Work out the finished part from the listing and answer in its coordinate system (mm). Face numbers are marked on the shaded views. A direction names the side the tool comes from. Give positions to 0.01 mm unless a question says otherwise; leave off trailing zeros. Write each loop counter-clockwise with the first axis right and the second up, starting at its lowest first coordinate (ties: lowest second). Pieces come first, ordered by that corner, then holes. Notation, with made-up numbers: (67, -28.75) -> (86, -28.75) arc R22 cw to (86, -8.75) -> close; hole circle Ø8 at (72.5, 68.25). An arc over 180 degrees is marked (long way). Use a Markdown table: item, result. Add a question column.
Q1. Section A-A, the plane x = 16.75 is taken. Give the vertices of the cut face in (y, z).
Q2. Consider line 1 (Y direction, x = 0.8, z = 10); line 2 (Y direction, x = 20.75, z = 20). Determine where each line is inside the solid, lowest interval first.
Q3. Each of these flat-tipped pins is pushed along its axis until it touches: pin 1 Ø1 at (x, z) = (19, 28) entering from +Y; pin 2 Ø9.5 at (y, z) = (11.5, 27) entering from +X. Where does it stop, or does it pass through?
Q4. For the marked faces 1 and 2, determine the directions among +Z, -Z, +X, -X, +Y, -Y from which every point of the face is accessible in a straight line to the end or side of a thin tool.
Q5. Section B-B, the plane z = 10 is taken. Give the vertices of the cut face in (x, y).
Q6. Section C-C, the plane y = 15 is taken. Give the vertices of the cut face in (x, z), plus the area to 3 significant figures.
Q7. Section D-D, the plane z = 30 is taken. Give the vertices of the cut face in (x, y).
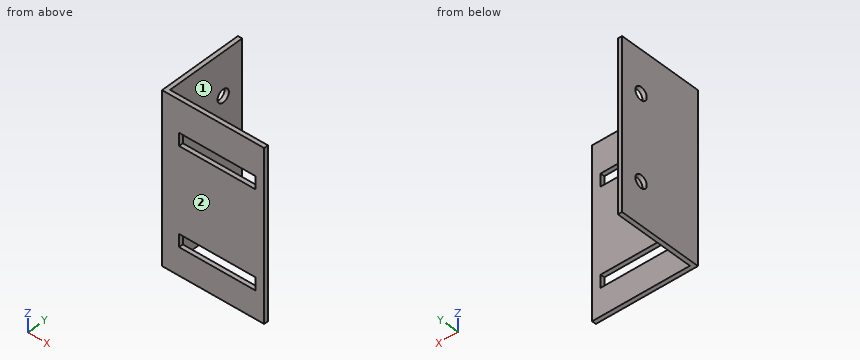
from build123d import *

# Parameters (mm, degrees)
BOSS_EXTRUDE1_DEPTH = 40
SKETCH2_W           = 18
SKETCH2_H           = 3
CUT_EXTRUDE1_DEPTH  = 10
SKETCH3_R           = 1.5
CUT_EXTRUDE2_DEPTH  = 10


with BuildPart() as part:
    # Sketch1 → Boss-Extrude1 (new body)
    with BuildSketch(Plane.XY):
        Polygon((0, 0), (24, 0), (24, 1), (1, 1), (1, 20), (0, 20), align=None)
    extrude(amount=BOSS_EXTRUDE1_DEPTH)

    # Sketch2 → Cut-Extrude1 (cut)
    with BuildSketch(Plane(origin=(0, 1, 0), x_dir=(1, 0, 0), z_dir=(0, 1, 0))):
        with Locations((13, -8)):
            Rectangle(SKETCH2_W, SKETCH2_H)
        with Locations((13, -31)):
            Rectangle(SKETCH2_W, SKETCH2_H)
    extrude(amount=-CUT_EXTRUDE1_DEPTH, mode=Mode.SUBTRACT)

    # Sketch3 → Cut-Extrude2 (cut)
    with BuildSketch(Plane.ZY):
        with Locations((30, 15)):
            Circle(SKETCH3_R)
        with Locations((10, 15)):
            Circle(SKETCH3_R)
    extrude(amount=-CUT_EXTRUDE2_DEPTH, mode=Mode.SUBTRACT)


solid = part.part
Result set:
| question | item | result |
|---|---|---|
| 1 | outline | (0, 0) -> (1, 0) -> (1, 6.5) -> (0, 6.5) -> close; (0, 9.5) -> (1, 9.5) -> (1, 29.5) -> (0, 29.5) -> close; (0, 32.5) -> (1, 32.5) -> (1, 40) -> (0, 40) -> close |
| 2 | line 1 | y = 0 to 13.5, 16.5 to 20 |
| 2 | line 2 | y = 0 to 1 |
| 3 | pin 1 | stops at y = 1 |
| 3 | pin 2 | stops at x = 1 |
| 4 | face 1 | +Z, -Z, +X, +Y |
| 4 | face 2 | +Z, -Z, +X, -X, -Y |
| 5 | outline | (0, 0) -> (24, 0) -> (24, 1) -> (1, 1) -> (1, 13.5) -> (0, 13.5) -> close; (0, 16.5) -> (1, 16.5) -> (1, 20) -> (0, 20) -> close |
| 6 | outline | (0, 0) -> (1, 0) -> (1, 8.5) -> (0, 8.5) -> close; (0, 11.5) -> (1, 11.5) -> (1, 28.5) -> (0, 28.5) -> close; (0, 31.5) -> (1, 31.5) -> (1, 40) -> (0, 40) -> close |
| 6 | area | 34.0 mm2 |
| 7 | outline | (0, 0) -> (4, 0) -> (4, 1) -> (1, 1) -> (1, 13.5) -> (0, 13.5) -> close; (0, 16.5) -> (1, 16.5) -> (1, 20) -> (0, 20) -> close; (22, 0) -> (24, 0) -> (24, 1) -> (22, 1) -> close |
